The figure shows three views and two pictorial views of one solid part (mm, origin at its lowest corner). Answer the questions. A direction names the side the tool comes from. Round coordinates to 2 decimals unless told otherwise and drop trailing zeros. Write each loop counter-clockwise with the first axis right and the second up, starting at its lowest first coordinate (ties: lowest second). Pieces come first, ordered by that corner, then holes.
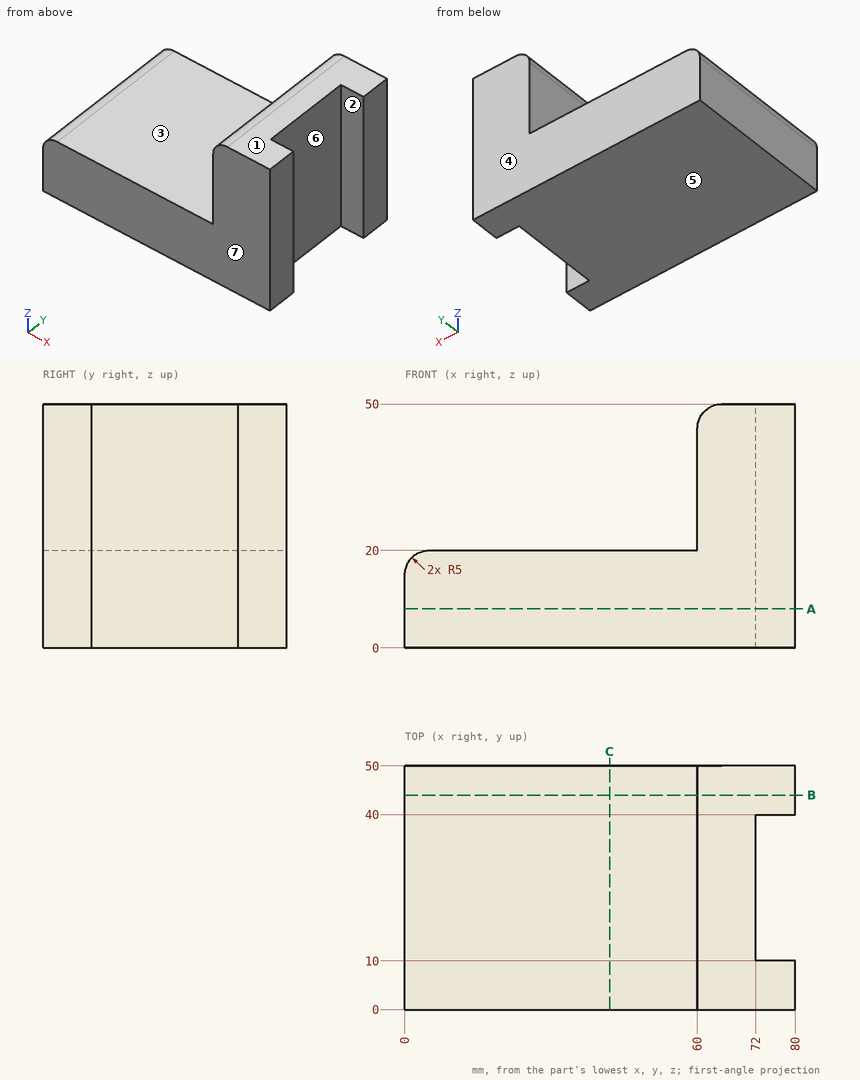
Q1. Determine the mould class of the marked faces 4, 5, 6 and 7 for opening direction Y: pulls with the +Y half, pulls with the -Y half, needs draft (parallel to the pull), parting line crosses it, or undercut.
Verdict:
face 4: pulls with the +Y half
face 5: needs draft
face 6: undercut
face 7: pulls with the -Y half
Q2. Section C-C (x = 42) is taken. Determine the outline of the cut face in (y, z).
Verdict:
outline: (0, 0) - (50, 0) - (50, 20) - (0, 20) - close
Q3. Straight lines are drawn through the part: probe 1 along X at (y, z) = (25, 7.5); probe 2 along Z at (x, y) = (18, 17); probe 3 along X at (y, z) = (44.5, 25.5). For each, find the intervals that lie inside material, in ascending order.
Verdict:
probe 1: x = 0 to 72
probe 2: z = 0 to 20
probe 3: x = 60 to 80
Q4. Which of the six approach directions +Z, -Z, +X, -X, +Y, -Y give full straight-line access (tool end or side, diameter ignored) to the marked faces 1, 2 and 3?
Verdict:
face 1: +Z, +X, -X, +Y, -Y
face 2: +Z, -Z, +X
face 3: +Z, -X, +Y, -Y
Q5. Flat-ended cylindrical pins translate along their axes: pin 1 Ø12.5 at (y, z) = (14.5, 33.5) entering from -X; pin 2 Ø4 at (x, y) = (60.5, 37) entering from +Z; pin 3 Ø5 at (x, z) = (55.5, 32.5) entering from +Y; pin 4 Ø2 at (y, z) = (24.5, 25.5) entering from +X. Find the tip coordinate at first contact, or state that the pin passes through.
Verdict:
pin 1: stops at x = 60
pin 2: stops at z = 49.33
pin 3: passes through
pin 4: stops at x = 72
Q6. Section A-A (z = 8) is taken. Determine the outline of the cut face in (x, y).
Verdict:
outline: (0, 0) - (80, 0) - (80, 10) - (72, 10) - (72, 40) - (80, 40) - (80, 50) - (0, 50) - close
Q7. Section B-B (y = 44) is taken. Determine the outline of the cut face in (x, z), then the cut area to 3 significant figures.
Verdict:
outline: (0, 0) - (80, 0) - (80, 50) - (65, 50) arc R5 ccw to (60, 45) - (60, 20) - (5, 20) arc R5 ccw to (0, 15) - close
area: 2,190 mm2
